Verification items for the finished model (mm, model axes). Face numbers are marked on the shaded views. Coordinates: 2 decimals unless noted, no trailing zeros. Order: outer loops, then holes, each group sorted by start corner. A loop starts at its lowest first (then second) coordinate and runs counter-clockwise, first axis right, second up.
Q1. Depth check by flat-ended pin: P1, Ø2.5, axis at x = 0, y = -7, coming from the -Z side; P2, Ø1, axis at y = 16.5, z = 1, coming from the +X side. Enter the tip coordinate at first touch or a pass-through.
Q2. Draft check along X on the marked faces 1, 2 and 3. Enter one of: pulls with the +X half, pulls with the -X half, needs draft (parallel to the pull), parting line crosses it, or undercut.
Q3. Cross-section at A-A, the plane x = 0. Record the boundary of the cut face in (y, z).
Q4. Cross-section at B-B, the plane z = 2.5. Count the separate pieces of the cut face and the enclosed holes in it, and give its area (3 significant figures).
Q5. Cross-section at C-C, the plane y = 0. Record the boundary of the cut face in (x, z).
Q6. Thickness scan on line 1 (Y direction, x = 0, z = 2); line 2 (X direction, y = -4, z = 2.35); line 3 (Y direction, x = -0.5, z = 0.5). Record the ranges inside material, lowest first.
Q7. Cross-section at D-D, the plane x = -16.5. Record the boundary of the cut face in (y, z), and give its area (3 significant figures).
from build123d import *

# Parameters (mm, degrees)
SKETCH_1_R      = 1.5
SKETCH_1_R_2    = 5
EXTRUDE_1_DEPTH = 3


with BuildPart() as part:
    # 草图1 → 凸台-拉伸1 (new body)
    with BuildSketch(Plane.XY):
        with BuildLine():
            Line((-2.598076211, 21.5), (-19.918584287, -8.5))
            ThreePointArc((-19.918584287, -8.5), (-19.918584287, -11.5), (-17.320508076, -13))
            Line((-17.320508076, -13), (17.320508076, -13))
            ThreePointArc((17.320508076, -13), (19.918584287, -11.5), (19.918584287, -8.5))
            Line((19.918584287, -8.5), (2.598076211, 21.5))
            ThreePointArc((2.598076211, 21.5), (0, 23), (-2.598076211, 21.5))
        make_face()
        with Locations((-17.320508076, -10)):
            Circle(SKETCH_1_R, mode=Mode.SUBTRACT)
        with Locations((0, 20)):
            Circle(SKETCH_1_R, mode=Mode.SUBTRACT)
        with Locations((17.320508076, -10)):
            Circle(SKETCH_1_R, mode=Mode.SUBTRACT)
        Circle(SKETCH_1_R_2, mode=Mode.SUBTRACT)
        with Locations((0, 7)):
            Circle(SKETCH_1_R, mode=Mode.SUBTRACT)
        with Locations((0, -7)):
            Circle(SKETCH_1_R, mode=Mode.SUBTRACT)
        with Locations((-7, 0)):
            Circle(SKETCH_1_R, mode=Mode.SUBTRACT)
        with Locations((7, 0)):
            Circle(SKETCH_1_R, mode=Mode.SUBTRACT)
    extrude(amount=EXTRUDE_1_DEPTH)


solid = part.part
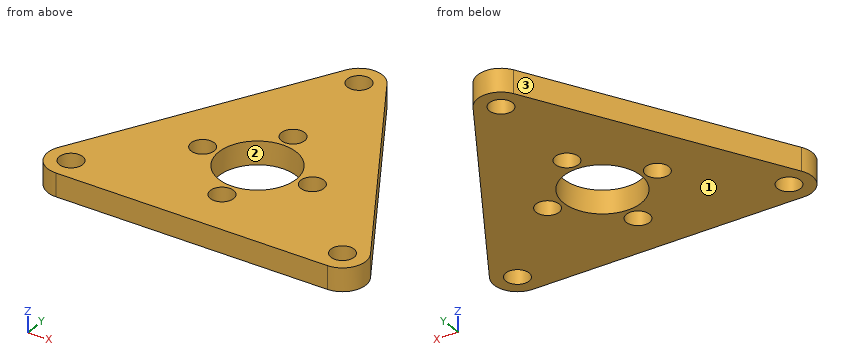
Check values:
1. P1: passes through
1. P2: stops at x = 5.77
2. face 1: needs draft
2. face 2: undercut
2. face 3: pulls with the -X half
3. outline: (-13, 0) - (-8.5, 0) - (-8.5, 3) - (-13, 3) - close; (-5.5, 0) - (-5, 0) - (-5, 3) - (-5.5, 3) - close; (5, 0) - (5.5, 0) - (5.5, 3) - (5, 3) - close; (8.5, 0) - (18.5, 0) - (18.5, 3) - (8.5, 3) - close; (21.5, 0) - (23, 0) - (23, 3) - (21.5, 3) - close
4. separate pieces: 1
4. enclosed holes: 8
4. area: 732 mm2
5. outline: (-15.01, 0) - (-8.5, 0) - (-8.5, 3) - (-15.01, 3) - close; (-5.5, 0) - (-5, 0) - (-5, 3) - (-5.5, 3) - close; (5, 0) - (5.5, 0) - (5.5, 3) - (5, 3) - close; (8.5, 0) - (15.01, 0) - (15.01, 3) - (8.5, 3) - close
6. line 1: y = -13 to -8.5, -5.5 to -5, 5 to 5.5, 8.5 to 18.5, 21.5 to 23
6. line 2: x = -17.32 to -3, 3 to 17.32
6. line 3: y = -13 to -8.41, -5.59 to -4.97, 4.97 to 5.59, 8.41 to 18.59, 21.41 to 22.96
7. outline: (-13, 0) - (-11.26, 0) - (-11.26, 3) - (-13, 3) - close; (-8.74, 0) - (-2.58, 0) - (-2.58, 3) - (-8.74, 3) - close
7. area: 23.7 mm2
